Part model, mm, in its own coordinate system. Face numbers are marked on the shaded views. A direction names the side the tool comes from. Give positions to 0.01 mm unless a question says otherwise; leave off trailing zeros. Write each loop counter-clockwise with the first axis right and the second up, starting at its lowest first coordinate (ties: lowest second). Pieces come first, ordered by that corner, then holes. Notation, with made-up numbers: M 81.25,-31.75 L 119.25,-31.75 A14 cw 119.25,-14.75 Z; hole C -6.5,18 d11. An arc over 180 degrees is marked long. Use a Markdown table: item, result. Add a question column.
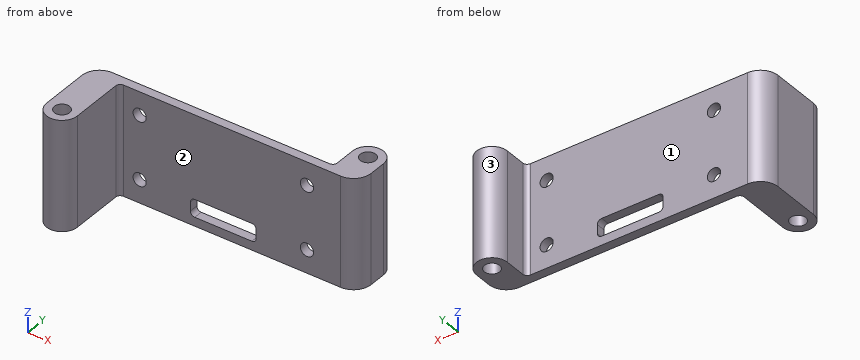
Autodesk Inventor part; units mm, degrees
ref_plane "YZ Plane" through (0, 0, 0) normal (1, 0, 0) x (0, 1, 0)
ref_plane "XZ Plane" through (0, 0, 0) normal (0, 1, 0) x (-1, 0, 0)
ref_plane "XY Plane" through (0, 0, 0) normal (0, 0, 1) x (1, 0, 0)
sketch "Skizze2" plane through (0, 0, 0) normal (0, 0, 1) x (1, 0, 0)
  line L0 (0, 0) -> (36.75, -63.6529) construction
  line L1 (0, 0) -> (73.5, 0) construction
  line L2 (36.75, -63.6529) -> (20.2955, -73.1529) construction
  line L3 (0, 0) -> (-34.202, -93.9693) construction
  line L4 (0, 0) -> (100, 0) construction
  circle A0 centre (-34.202, -93.9693) radius 1.75
  circle A1 centre (20.2955, -73.1529) radius 1.75
  arc A2 (-37.702, -93.9693) -> (-30.702, -93.9693) centre (-34.202, -93.9693) ccw
  arc A3 (23.7955, -73.1529) -> (16.7955, -73.1529) centre (20.2955, -73.1529) ccw
  line L5 (-37.702, -93.9693) -> (-37.702, -78.9693)
  line L6 (-37.702, -78.9693) -> (16.7955, -78.9693)
  line L7 (16.7955, -78.9693) -> (16.7955, -73.1529)
  line L8 (23.7955, -73.1529) -> (23.7955, -80.9693)
  line L9 (23.7955, -80.9693) -> (-30.702, -80.9693)
  line L10 (-30.702, -80.9693) -> (-30.702, -93.9693)
  line L11 (-30.702, -93.9693) -> (-37.702, -93.9693) construction
  line L12 (16.7955, -73.1529) -> (23.7955, -73.1529) construction
  dimension "d16" = 73.5
  dimension "d17" = 60
  dimension "d18" = 19
  dimension "d19" = 100
  dimension "d20" = 110
  dimension "d21" = 3.5
  dimension "d22" = 7
  dimension "d23" = 2
  dimension "d24" = 13
extrude "Extrusion2" add sketch "Skizze2" along normal blind 25
sketch "Skizze3" plane through (-30.702, -80.9693, 0) normal (0, -1, 0) x (1, 0, 0)
  line L0 (4.6988, 19.739) -> (42.7988, 19.739) construction
  line L1 (42.7988, 19.739) -> (42.7988, 5.261) construction
  line L2 (42.7988, 5.261) -> (4.6988, 5.261) construction
  line L3 (4.6988, 5.261) -> (4.6988, 19.739) construction
  line L4 (0, 0) -> (0, 25) construction
  line L5 (0, 12.5) -> (47.4975, 12.5) construction
  line L6 (47.4975, 0) -> (47.4975, 25) construction
  line L7 (0, 25) -> (54.4975, 25) construction
  line L8 (23.7488, 25) -> (23.7488, 0) construction
  line L9 (0, 0) -> (54.4975, 0) construction
  circle A0 centre (42.7988, 19.739) radius 1.5
  circle A1 centre (4.6988, 5.261) radius 1.5
  line L10 (2.1588, 22.4949) -> (45.3388, 22.4949) construction
  line L11 (45.3388, 22.4949) -> (45.3388, 2.5051) construction
  line L12 (45.3388, 2.5051) -> (2.1588, 2.5051) construction
  line L13 (2.1588, 2.5051) -> (2.1588, 22.4949) construction
  line L14 (16.2488, 2.0051) -> (31.2488, 2.0051)
  line L15 (31.2488, 2.0051) -> (31.2488, 6.0051)
  line L16 (31.2488, 6.0051) -> (16.2488, 6.0051)
  line L17 (16.2488, 6.0051) -> (16.2488, 2.0051)
  circle A2 centre (4.6988, 19.739) radius 1.5
  circle A3 centre (42.7988, 5.261) radius 1.5
  point P0 (30.702, 0)
  point P1 (23.7488, 12.5)
  point P2 (23.7488, 19.739)
  point P3 (42.7988, 12.5)
  point P4 (23.7488, 22.4949)
  point P5 (45.3388, 12.5)
  point P6 (23.7488, 6.0051)
  dimension "d27" = 38.1
  dimension "d28" = 14.478
  dimension "d29" = 3
  dimension "d30" = 43.18
  dimension "d31" = 19.9898
  dimension "d32" = 15
  dimension "d33" = 4
  dimension "d39" = 0.5
extrude "Extrusion3" cut sketch "Skizze3" against normal up to next
fillet "Rundung1" radius 1 4 edges at (-14.4532, -79.9693, 2.0051) (-14.4532, -79.9693, 6.0051) (0.5468, -79.9693, 2.0051) (0.5468, -79.9693, 6.0051)
fillet "Rundung2" radius 4 2 edges at (23.7955, -80.9693, 12.5) (-37.702, -78.9693, 12.5)
fillet "Rundung3" radius 1 2 edges at (16.7955, -78.9693, 12.5) (-30.702, -80.9693, 12.5)
properties part number "US Halterung rechts" material "ABS-Kunststoff"
1. Cut at B-B (x = 11.5). Write the cut outline in (y, z).
2. Flat gauge pins, fed straight in: pin 1 (1 mm diameter, centred on x = -4.5, y = -80, fed in from -Z); pin 2 (1.6 mm diameter, centred on y = -80, z = 4, fed in from +X); pin 3 (1 mm diameter, centred on x = 1.5, z = 14, fed in from -Y); pin 4 (2 mm diameter, centred on y = -80.5, z = 4.5, fed in from -X). Where does each tip first touch, or does it go through?
3. Drill centre lines: probe 1 along Z at (x, y) = (12, -79); probe 2 along Y at (x, z) = (-34.5, 8.25); probe 3 along Y at (x, z) = (-21, 21.25). Where is each one in solid material? Low to high. Write a range as [from, to].
4. Cut at A-A (z = 15.5). Write the cut outline in (x, y).
5. Cut at C-C (y = -74.25). Write the cut outline in (x, z), then the cut area to 3 significant figures.
6. Cut at D-D (y = -80). Write the cut outline in (x, z), then the cut area to 3 significant figures.
7. Tool access for the marked faces 1, 2 and 3: list every direction of +Z, -Z, +X, -X, +Y, -Y with a clear straight run to the whole face (end or side of a thin tool).
A:
| question | item | result |
|---|---|---|
| 1 | outline | M -80.97,0 L -78.97,0 L -78.97,3.88 L -80.97,3.88 Z; M -80.97,6.64 L -78.97,6.64 L -78.97,18.36 L -80.97,18.36 Z; M -80.97,21.12 L -78.97,21.12 L -78.97,25 L -80.97,25 Z |
| 2 | pin 1 | stops at z = 0 |
| 2 | pin 2 | stops at x = 23.12 |
| 2 | pin 3 | stops at y = -80.97 |
| 2 | pin 4 | stops at x = -37.42 |
| 3 | probe 1 | z = [0, 3.76], [6.76, 18.24], [21.24, 25] |
| 3 | probe 2 | y = [-97.46, -95.69], [-92.24, -79.05] |
| 3 | probe 3 | y = [-80.97, -78.97] |
| 4 | outline | M -37.7,-93.97 A3.5 ccw -30.7,-93.97 L -30.7,-81.97 A1 cw -29.7,-80.97 L 19.8,-80.97 A4 ccw 23.8,-76.97 L 23.8,-73.15 A3.5 ccw 16.8,-73.15 L 16.8,-77.97 A1 cw 15.8,-78.97 L -33.7,-78.97 A4 ccw -37.7,-82.97 Z; hole C -34.2,-93.97 d3.5; hole C 20.3,-73.15 d3.5 |
| 5 | outline | M 16.8,0 L 18.93,0 L 18.93,25 L 16.8,25 Z; M 21.66,0 L 23.8,0 L 23.8,25 L 21.66,25 Z |
| 5 | area | 107 mm² |
| 6 | outline | M -36.38,0 L 22.41,0 L 22.41,25 L -36.38,25 Z; hole C -26,5.26 d3; hole C -26,19.74 d3; hole M -14.45,3.01 A1 ccw -13.45,2.01 L -0.45,2.01 A1 ccw 0.55,3.01 L 0.55,5.01 A1 ccw -0.45,6.01 L -13.45,6.01 A1 ccw -14.45,5.01 Z; hole C 12.1,5.26 d3; hole C 12.1,19.74 d3 |
| 6 | area | 1,380 mm² |
| 7 | face 1 | +Z, -Z, -X, +Y |
| 7 | face 2 | +Z, -Z, +X, -Y |
| 7 | face 3 | +Z, -Z, +Y |
